Verification items for the finished model (mm, model axes). Face numbers are marked on the shaded views. A direction names the side the tool comes from. Round coordinates to 2 decimals unless told otherwise and drop trailing zeros. Order: outer loops, then holes, each group sorted by start corner. A loop starts at its lowest first (then second) coordinate and runs counter-clockwise, first axis right, second up. Notation, with made-up numbers: M -37.75,-5.5 L 15.25,-5.5 A20 ccw 15.25,13.5 Z; hole C 2,6 d4. An arc over 180 degrees is marked long. Use CSV: the item, a comma, the result in double quotes. Start each with the question number.
Q1. Sectioned sample at A-A (z = 5.75). Enter the section's corners in (x, y).
Q2. Scan lines: line 1 (X direction, y = 20, z = 6.5); line 2 (Z direction, x = -30, y = 14.5); line 3 (X direction, y = -28, z = 8.75). Record each from-to range of solid material in increasing order.
Q3. Mould release check, pull along X, two halves, no side actions. Record for the marked faces 3, 4, 5 and 6: +X half, -X half, draft (parallel to the pull), parting line (faces both ways), or undercut.
Q4. Sectioned sample at B-B (y = -6). Enter the section's corners in (x, z), and give its area (3 significant figures).
Q5. Set-up check for the marked faces 1 and 2: record each of +Z, -Z, +X, -X, +Y, -Y from which the full face is reachable in a straight line by a thin tool's end or side.
Q6. Gauge pin test, flat ends, axial feed: pin 1 Ø6 at (y, z) = (-32.5, 2) entering from -X; pin 2 Ø6 at (y, z) = (47, 4.5) entering from -X; pin 3 Ø1 at (x, z) = (-13, 5.5) entering from -Y. Record the tip position at first contact, or that the pin passes through.
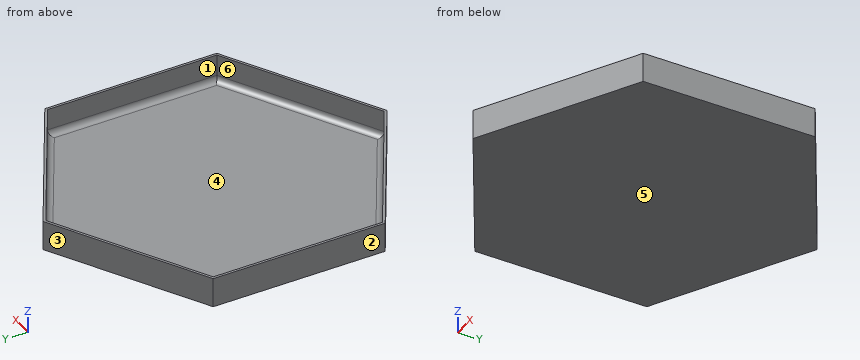
```python
from build123d import *

# Parameters (mm, degrees)
F1_DEPTH = 10
F2_T     = -0.8
F3_R     = 2


with BuildPart() as f1:
    # F0 (on Top) → F1 (new body)
    with BuildSketch(Plane.XY):
        Polygon((53.4592177784, 30.4124803951), (3.4592177784, 59.2799938546), (-46.5407822216, 30.4124803951), (-46.5407822216, -27.3225465238), (3.4592177784, -56.1900599833), (53.4592177784, -27.3225465238), align=None)
    extrude(amount=F1_DEPTH)

    # F2
    f2_openings = [f1.faces().sort_by_distance(p)[0] for p in [
        (3.459218, 1.544967, 10),
    ]]
    offset(amount=F2_T, openings=f2_openings)

    # F3
    f3_edges = [f1.edges().sort_by_distance(p)[0] for p in [
        (28.059218, -41.063483, 0.8),
        (52.659218, 1.544967, 0.8),
        (28.059218, 44.153417, 0.8),
        (-21.140782, 44.153417, 0.8),
        (-45.740782, 1.544967, 0.8),
        (-21.140782, -41.063483, 0.8),
    ]]
    fillet(f3_edges, radius=F3_R)


solid = f1.part
```
Verdict:
1,outline,"M -46.54,-27.32 L 3.46,-56.19 L 53.46,-27.32 L 53.46,30.41 L 3.46,59.28 L -46.54,30.41 Z; hole M -45.74,-26.86 L 3.46,-55.27 L 52.66,-26.86 L 52.66,29.95 L 3.46,58.36 L -45.74,29.95 Z"
2,line 1,"x = -46.54 to -45.74, 52.66 to 53.46"
2,line 2,"z = 0 to 0.8"
2,line 3,"x = -45.37 to -43.77, 50.69 to 52.29"
3,face 3,"-X half"
3,face 4,"undercut"
3,face 5,"draft"
3,face 6,"undercut"
4,outline,"M -46.54,0 L 53.46,0 L 53.46,10 L 52.66,10 L 52.66,2.8 A2 cw 50.66,0.8 L -43.74,0.8 A2 cw -45.74,2.8 L -45.74,10 L -46.54,10 Z"
4,area,"96.4 mm²"
5,face 1,"+Z"
5,face 2,"+Z, -Z, -X, +Y, -Y"
6,pin 1,"stops at x = -42.77"
6,pin 2,"stops at x = -23.01"
6,pin 3,"stops at y = -46.98"
